Geometry check sheet. Reference: drawing and pictorial views, mm from the part's lowest x, y, z. Give positions to 0.01 mm unless a question says otherwise; leave off trailing zeros. Order: outer loops, then holes, each group sorted by start corner. A loop starts at its lowest first (then second) coordinate and runs counter-clockwise, first axis right, second up. Notation, with made-up numbers: M -29,14.25 L 21,14.25 A17 ccw 21,37.25 Z; hole C 88.5,89 d7. An arc over 180 degrees is marked long. Answer as CSV lines item,"result". Start each with the question number.
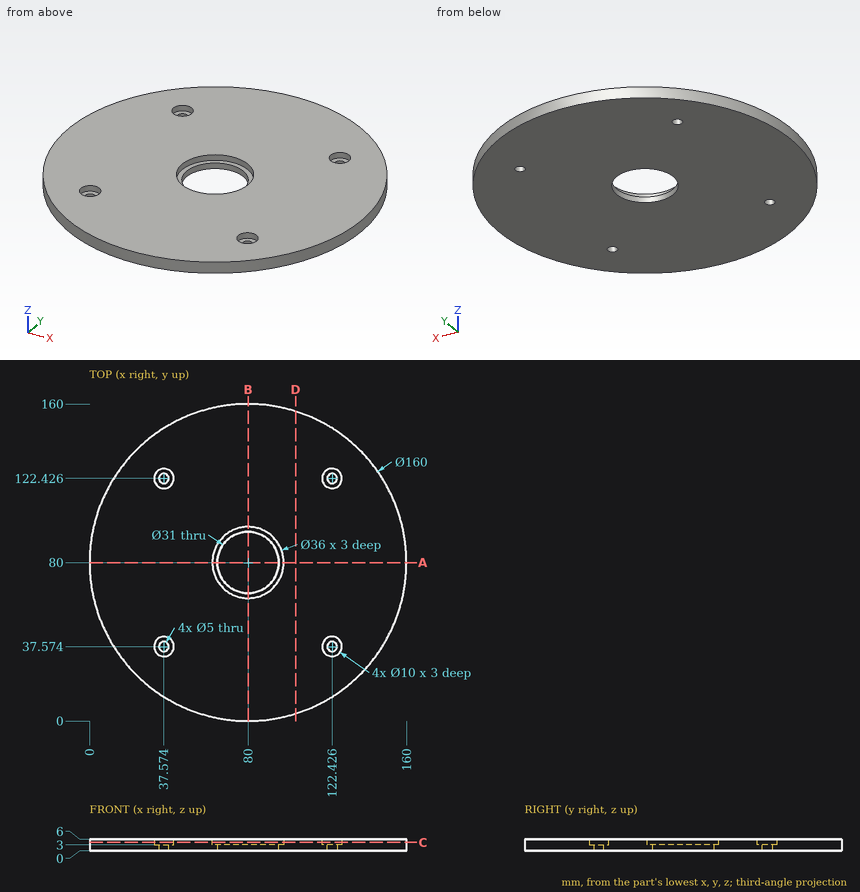
Item 1: Section check D-D on x = 104. Record the boundary of the cut face in (y, z) (1 decimal).
Item 2: Scan lines: line 1 along Y through (x, z) = (121, 2.75) (1 decimal); line 2 along Y through (x, z) = (80, 4.6); line 3 along X through (y, z) = (71, 3.2). Record each from-to range of solid material in increasing order.
Item 3: Section check C-C on z = 4.25. Record the boundary of the cut face in (x, y).
Item 4: Depth check by flat-ended pin: pin 1 Ø10 at (x, y) = (42.5, 136.5) entering from -Z; pin 2 Ø3 at (y, z) = (118.5, 5) entering from +X; pin 3 Ø1 at (x, z) = (21, 1) entering from +Y; pin 4 Ø3 at (x, y) = (39, 38.5) entering from +Z. Enter the tip coordinate at first touch or a pass-through.
Item 5: Section check A-A on y = 80. Record the boundary of the cut face in (x, z), then the cut area to 3 significant figures.
Numbers:
1,outline,"M 3.7,0 L 156.3,0 L 156.3,6 L 3.7,6 Z"
2,line 1,"11.3 to 35.5, 39.6 to 120.4, 124.5 to 148.7"
2,line 2,"0 to 62, 98 to 160"
2,line 3,"0.51 to 64.41, 95.59 to 159.49"
3,outline,"C 80,80 d160; hole C 37.57,37.57 d10; hole C 37.57,122.43 d10; hole C 80,80 d36; hole C 122.43,37.57 d10; hole C 122.43,122.43 d10"
4,pin 1,"z = 0"
4,pin 2,"x = 150.93"
4,pin 3,"y = 134.57"
4,pin 4,"z = 3"
5,outline,"M 0,0 L 64.5,0 L 64.5,3 L 62,3 L 62,6 L 0,6 Z; M 95.5,0 L 160,0 L 160,6 L 98,6 L 98,3 L 95.5,3 Z"
5,area,"759 mm2"
